Geometry: final body of the model. Coordinates: model frame, mm. Give positions to 0.01 mm unless a question says otherwise; leave off trailing zeros. Order: outer loops, then holes, each group sorted by start corner. A loop starts at its lowest first (then second) coordinate and runs counter-clockwise, first axis right, second up. Notation, with made-up numbers: (7, 27.5) -> (58, 27.5) arc R19 cw to (58, 44.5) -> close; hole circle Ø7 at (46, 25). An arc over 180 degrees is marked (long way). Answer in a Markdown table with one row per item. Add a question column.
Q1. Cut plane A-A on x = -33. Return the cut outline in (y, z), and give its area (3 significant figures).
Q2. Cut plane B-B on z = -32. Return the cut outline in (x, y).
Q3. Line query: line 1 along X through (y, z) = (2.45, -75); line 2 along Z through (x, y) = (41, 1.6). Output: solid intervals per line, ascending. Write a range as from..to.
Q4. Cut plane C-C on y = 2.3. Count the separate pieces of the cut face and the enclosed holes in it, and give its area (3 significant figures).
from build123d import *

# Parameters (mm, degrees)
SKETCH1_W           = 400
SKETCH1_H           = 300
BOSS_EXTRUDE2_DEPTH = 3
SKETCH5_W           = 3
SKETCH5_H           = 27
CUT_EXTRUDE4_DEPTH  = 3
SKETCH6_W           = 3
SKETCH6_H           = 27
CUT_EXTRUDE5_DEPTH  = 3
SKETCH12_W          = 27
SKETCH12_H          = 3
CUT_EXTRUDE10_DEPTH = 10
SKETCH13_W          = 27
SKETCH13_H          = 3
CUT_EXTRUDE11_DEPTH = 10


with BuildPart() as part:
    # Sketch1 → Boss-Extrude2 (new body)
    with BuildSketch(Plane(origin=(0, 0, 0), x_dir=(1, 0, 0), z_dir=(0, 1, 0))):
        Rectangle(SKETCH1_W, SKETCH1_H)
    extrude(amount=BOSS_EXTRUDE2_DEPTH)

    # Sketch5 → Cut-Extrude4 (cut)
    with BuildSketch(Plane(origin=(0, 3, 0), x_dir=(1, 0, 0), z_dir=(0, 1, 0))):
        with Locations((-188.5, 126.5)):
            Rectangle(SKETCH5_W, SKETCH5_H)
        with Locations((-188.5, 76.5)):
            Rectangle(SKETCH5_W, SKETCH5_H)
        with Locations((-188.5, 26.5)):
            Rectangle(SKETCH5_W, SKETCH5_H)
        with Locations((-188.5, -23.5)):
            Rectangle(SKETCH5_W, SKETCH5_H)
        with Locations((-188.5, -73.5)):
            Rectangle(SKETCH5_W, SKETCH5_H)
        with Locations((-188.5, -123.5)):
            Rectangle(SKETCH5_W, SKETCH5_H)
    extrude(amount=-CUT_EXTRUDE4_DEPTH, mode=Mode.SUBTRACT)

    # Sketch6 → Cut-Extrude5 (cut)
    with BuildSketch(Plane(origin=(0, 3, 0), x_dir=(1, 0, 0), z_dir=(0, 1, 0))):
        with Locations((188.5, 126.5)):
            Rectangle(SKETCH6_W, SKETCH6_H)
        with Locations((188.5, 76.5)):
            Rectangle(SKETCH6_W, SKETCH6_H)
        with Locations((188.5, 26.5)):
            Rectangle(SKETCH6_W, SKETCH6_H)
        with Locations((188.5, -23.5)):
            Rectangle(SKETCH6_W, SKETCH6_H)
        with Locations((188.5, -73.5)):
            Rectangle(SKETCH6_W, SKETCH6_H)
        with Locations((188.5, -123.5)):
            Rectangle(SKETCH6_W, SKETCH6_H)
    extrude(amount=-CUT_EXTRUDE5_DEPTH, mode=Mode.SUBTRACT)

    # Sketch12 → Cut-Extrude10 (cut)
    with BuildSketch(Plane.XZ):
        with Locations((-176.5, -144.5)):
            Rectangle(SKETCH12_W, SKETCH12_H)
        with Locations((-105.9, -144.5)):
            Rectangle(SKETCH12_W, SKETCH12_H)
        with Locations((-35.3, -144.5)):
            Rectangle(SKETCH12_W, SKETCH12_H)
        with Locations((35.3, -144.5)):
            Rectangle(SKETCH12_W, SKETCH12_H)
        with Locations((105.9, -144.5)):
            Rectangle(SKETCH12_W, SKETCH12_H)
        with Locations((176.5, -144.5)):
            Rectangle(SKETCH12_W, SKETCH12_H)
    extrude(amount=-CUT_EXTRUDE10_DEPTH, mode=Mode.SUBTRACT)

    # Sketch13 → Cut-Extrude11 (cut)
    with BuildSketch(Plane(origin=(0, 0, 0), x_dir=(-1, 0, 0), z_dir=(0, -1, 0))):
        with Locations((176.5, -144.5)):
            Rectangle(SKETCH13_W, SKETCH13_H)
        with Locations((105.9, -144.5)):
            Rectangle(SKETCH13_W, SKETCH13_H)
        with Locations((35.3, -144.5)):
            Rectangle(SKETCH13_W, SKETCH13_H)
        with Locations((-35.3, -144.5)):
            Rectangle(SKETCH13_W, SKETCH13_H)
        with Locations((-105.9, -144.5)):
            Rectangle(SKETCH13_W, SKETCH13_H)
        with Locations((-176.5, -144.5)):
            Rectangle(SKETCH13_W, SKETCH13_H)
    extrude(amount=-CUT_EXTRUDE11_DEPTH, mode=Mode.SUBTRACT)


solid = part.part
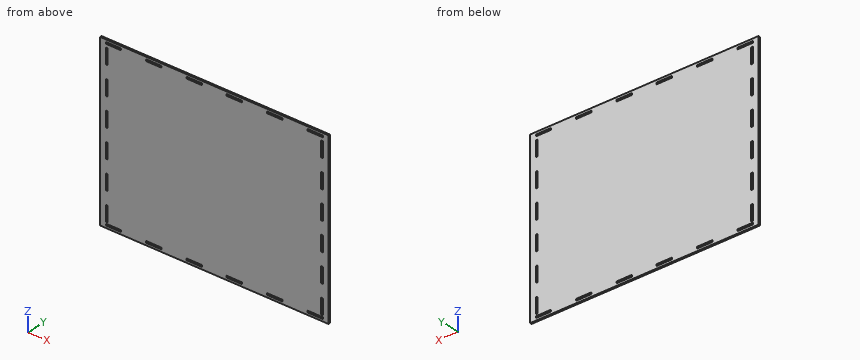
Completed:
| question | item | result |
|---|---|---|
| 1 | outline | (0, -150) -> (3, -150) -> (3, -146) -> (0, -146) -> close; (0, -143) -> (3, -143) -> (3, 143) -> (0, 143) -> close; (0, 146) -> (3, 146) -> (3, 150) -> (0, 150) -> close |
| 1 | area | 882 mm² |
| 2 | outline | (-200, 0) -> (-190, 0) -> (-190, 3) -> (-200, 3) -> close; (-187, 0) -> (187, 0) -> (187, 3) -> (-187, 3) -> close; (190, 0) -> (200, 0) -> (200, 3) -> (190, 3) -> close |
| 3 | line 1 | x = -200..-190, -187..187, 190..200 |
| 3 | line 2 | z = -150..-146, -143..143, 146..150 |
| 4 | separate pieces | 1 |
| 4 | enclosed holes | 24 |
| 4 | area | 118,000 mm² |
